Design review of the part built by this model. Coordinates are the model's own, in mm. A direction names the side the tool comes from. Round coordinates to 2 decimals unless told otherwise and drop trailing zeros. Order: outer loops, then holes, each group sorted by start corner. A loop starts at its lowest first (then second) coordinate and runs counter-clockwise, first axis right, second up. Notation, with made-up numbers: (-16.5, -9) - (37.5, -9) arc R32 cw to (37.5, 17) - close; hole circle Ø1 at (-26.75, -3.75). An arc over 180 degrees is marked (long way). Use CSV: the item, a comma, the result in double quotes. Start each with the question number.
from build123d import *

# Parameters (mm, degrees)
SKETCH_1_R      = 7.5
EXTRUDE_1_DEPTH = 5
SKETCH_2_R      = 6
EXTRUDE_2_DEPTH = 130
SKETCH_3_R      = 4
EXTRUDE_3_DEPTH = 2.5
EXTRUDE_START   = -10
SKETCH_4_R      = 7.5
EXTRUDE_4_DEPTH = 10


with BuildPart() as part:
    # 草圖1 → 填料-伸長1 (new body)
    with BuildSketch(Plane(origin=(0, 0, 0), x_dir=(1, 0, 0), z_dir=(0, 1, 0))):
        with Locations(Location((0, 0, 0), (0, 0, 270))):
            Circle(SKETCH_1_R)
    extrude(amount=EXTRUDE_1_DEPTH)

    # 草圖2 → 填料-伸長2 (add)
    with BuildSketch(Plane(origin=(0, 5, 0), x_dir=(1, 0, 0), z_dir=(0, 1, 0))):
        with Locations(Location((0, 0, 0), (0, 0, 270))):
            Circle(SKETCH_2_R)
    extrude(amount=EXTRUDE_2_DEPTH)

    # 草圖3 → 填料-伸長3 (add, symmetric)
    with BuildSketch(Plane(origin=(0, 0, 0), x_dir=(0, 0, -1), z_dir=(1, 0, 0))):
        with BuildLine():
            Line((-7, 151), (-7, 135))
            Line((-7, 135), (7, 135))
            Line((7, 135), (7, 151))
            ThreePointArc((7, 151), (0, 158), (-7, 151))
        make_face()
        with Locations((0, 151)):
            Circle(SKETCH_3_R, mode=Mode.SUBTRACT)
    extrude(amount=EXTRUDE_3_DEPTH, both=True)

    # 草圖4 → 填料-伸長4 (add)
    with BuildSketch(Plane(origin=(0, 135, 0), x_dir=(1, 0, 0), z_dir=(0, 1, 0)).offset(EXTRUDE_START)):
        with Locations(Location((0, 0, 0), (0, 0, 270))):
            Circle(SKETCH_4_R)
    extrude(amount=EXTRUDE_4_DEPTH)


solid = part.part
Q1. Take a section at A-A (z = 0). State the section outline as (x, y) points, plus the area to 3 significant figures.
Q2. The part is to be moulded in two halves that separate along Y. For faces 1 (the flat face through (6, 5, 2)), 2 (the cylindrical face through (0, 158, 0)), 3 (the flat face through (2.5, 144, 0)), say which applies: +Y half, -Y half, draft (parallel to the pull), parting line (faces both ways), or undercut.
Q3. Take a section at D-D (y = 141). State the section outline as (x, z) points.
Q4. Clearance check with flat-ended pins moving along their axes: pin 1 (5 mm diameter, centred on x = -5.5, y = 120.5, fed in from +Z); pin 2 (1.5 mm diameter, centred on x = 0, y = 145.5, fed in from -Z); pin 3 (4 mm diameter, centred on x = 4, y = 72, fed in from +Z); pin 4 (7 mm diameter, centred on y = 151, z = 0, fed in from +X). State where each tip first meets the part, or that it passes through.
Q5. Take a section at C-C (y = 75.5). State the section outline as (x, z) points.
Q6. Take a section at B-B (x = 0). State the section outline as (y, z) points.
Q7. Tool access review of faces 4 (the flat face through (6, 125, 2)), 5 (the flat face through (0, 143, 7)), 6 (the flat face through (-2.5, 144, 0)), 7 (the flat face through (0, 143, -7)): name each direction out of +Z, -Z, +X, -X, +Y, -Y from which nothing blocks a thin tool from reaching the whole face with its end or side.
Q8. For L1, parallel to Y at x = -0.4, z = 0; L2, parallel to Y at x = 3.75, z = 1.75; L3, parallel to Z at x = 2.75, y = 133.5, list the stretches that pass through material, from the lowest coordinate up. Write a range as [from, to].
Findings below:
1,outline,"(-7.5, 0) - (7.5, 0) - (7.5, 5) - (6, 5) - (6, 125) - (7.5, 125) - (7.5, 135) - (2.5, 135) - (2.5, 147) - (-2.5, 147) - (-2.5, 135) - (-7.5, 135) - (-7.5, 125) - (-6, 125) - (-6, 5) - (-7.5, 5) - close; (-2.5, 155) - (2.5, 155) - (2.5, 158) - (-2.5, 158) - close"
1,area,"1,740 mm^2"
2,face 1,"undercut"
2,face 2,"+Y half"
2,face 3,"draft"
3,outline,"(-2.5, -7) - (2.5, -7) - (2.5, 7) - (-2.5, 7) - close"
4,pin 1,"stops at z = 5.2"
4,pin 2,"stops at z = -7"
4,pin 3,"stops at z = 5.66"
4,pin 4,"passes through"
5,outline,"circle Ø12 at (0, 0)"
6,outline,"(0, -7.5) - (5, -7.5) - (5, -6) - (125, -6) - (125, -7.5) - (135, -7.5) - (135, -7) - (151, -7) arc R7 ccw to (151, 7) - (135, 7) - (135, 7.5) - (125, 7.5) - (125, 6) - (5, 6) - (5, 7.5) - (0, 7.5) - close; hole circle Ø8 at (151, 0)"
7,face 4,"none"
7,face 5,"+Z, +X, -X, +Y"
7,face 6,"+Z, -Z, -X, +Y"
7,face 7,"-Z, +X, -X, +Y"
8,L1,"y = [0, 147], [155, 158]"
8,L2,"y = [0, 135]"
8,L3,"z = [-6.98, 6.98]"
